```python
from build123d import *

# Parameters (mm, degrees)
EXTRUDE_1_DEPTH     = 5
CUT_EXTRUDE_1_REACH = 82.779
SKETCH_2_R          = 1.5


with BuildPart() as part:
    # 草图1 → 凸台-拉伸1 (new body)
    with BuildSketch(Plane(origin=(0, 0, 0), x_dir=(1, 0, 0), z_dir=(0, 1, 0))):
        with BuildLine():
            Line((61.023746461, 33.569203074), (60.837080184, 37.600567015))
            Line((60.837080184, 37.600567015), (70.826313722, 38.06310353))
            Line((70.826313722, 38.06310353), (71.011329506, 34.067384676))
            ThreePointArc((71.011329506, 34.067384676), (49.082411457, -9.842070835), (0.164945446, -13.841976975))
            ThreePointArc((0.164945446, -13.841976975), (-2.286053035, -7.209284728), (4.346639213, -4.758286247))
            ThreePointArc((4.346639213, -4.758286247), (43.480612021, -1.558361335), (61.023746461, 33.569203074))
        make_face()
    extrude(amount=EXTRUDE_1_DEPTH)

    # 草图2 → 切除-拉伸1 (cut, up to next)
    with BuildSketch(Plane(origin=(0, 5, 0), x_dir=(1, 0, 0), z_dir=(0, 1, 0)), mode=Mode.PRIVATE) as cut_extrude_1_sk1:
        with Locations(Location((16.930413815, -13.232401329, 0), (0, 0, 270))):
            Circle(SKETCH_2_R)
    cut_extrude_1_tool1 = extrude(cut_extrude_1_sk1.sketch, amount=-CUT_EXTRUDE_1_REACH, mode=Mode.PRIVATE) & part.part
    # 草图2 → 切除-拉伸1 (cut, up to next)
    with BuildSketch(Plane(origin=(0, 5, 0), x_dir=(1, 0, 0), z_dir=(0, 1, 0)), mode=Mode.PRIVATE) as cut_extrude_1_sk2:
        with Locations(Location((41.522785914, -8.508722595, 0), (0, 0, 270))):
            Circle(SKETCH_2_R)
    cut_extrude_1_tool2 = extrude(cut_extrude_1_sk2.sketch, amount=-CUT_EXTRUDE_1_REACH, mode=Mode.PRIVATE) & part.part
    add(cut_extrude_1_tool1.solids().sort_by_distance((16.930414, 5, 13.232401))[0], mode=Mode.SUBTRACT)
    add(cut_extrude_1_tool2.solids().sort_by_distance((41.522786, 5, 8.508723))[0], mode=Mode.SUBTRACT)


solid = part.part
```
Input: part model. Units: mm. Frame: model coordinates. A direction names the side the tool comes from. Give positions to 0.01 mm unless a question says otherwise; leave off trailing zeros. Order: outer loops, then holes, each group sorted by start corner. A loop starts at its lowest first (then second) coordinate and runs counter-clockwise, first axis right, second up. Notation, with made-up numbers: (-36.5, 27.25) - (12.5, 27.25) arc R16 ccw to (12.5, 33.25) - close; hole circle Ø11 at (13, 58.25). An arc over 180 degrees is marked (long way). Use a Markdown table: item, result.
(1) Section query A-A (y = 3.85). Output: boundary loops of the cut face in (x, z).
Computed values:
| item | result |
|---|---|
| outline | (0.16, 13.84) arc R5 ccw to (4.35, 4.76) arc R40 cw to (61.02, -33.57) - (60.84, -37.6) - (70.83, -38.06) - (71.01, -34.07) arc R50 ccw to start; hole circle Ø3 at (16.93, 13.23); hole circle Ø3 at (41.52, 8.51) |
(2) Draft query along X for faces 1 (the flat face through (45, 5, 1)), 2 (the cylindrical face through (18.195, 2.535, 14.039)), 3 (the flat face through (65.76, 2.46, -37.83)). Return one class per face: released by +X, released by -X, zero draft, split by the parting line, or undercut.
Computed values:
| item | result |
|---|---|
| face 1 | zero draft |
| face 2 | undercut |
| face 3 | released by -X |
(3) Pin query (flat end, axial travel): pin 1 (2 mm diameter, centred on x = 27, y = 1, fed in from +Z). Return the tip coordinate at first contact, or that it passes through.
Computed values:
| item | result |
|---|---|
| pin 1 | stops at z = 18.18 |
(4) Section query B-B (z = 1.5). Output: boundary loops of the cut face in (x, y), then the cut area to 3 significant figures.
Computed values:
| item | result |
|---|---|
| outline | (43.57, 0) - (58.57, 0) - (58.57, 5) - (43.57, 5) - close |
| area | 75.0 mm2 |
(5) Access query for faces 4 (the flat face through (70.918, 2.465, -36.093)), 5 (the flat face through (60.93, 2.46, -35.56)). Directions: +Z, -Z, +X, -X, +Y, -Y. A direction counts if a zero-diameter tool reaches every point of the face in a straight line with its end or side. Return the directions, or none.
Computed values:
| item | result |
|---|---|
| face 4 | -Z, +X, +Y, -Y |
| face 5 | -X, +Y, -Y |
(6) Section query C-C (x = 7). Output: boundary loops of the cut face in (y, z), then the cut area to 3 significant figures.
Computed values:
| item | result |
|---|---|
| outline | (0, 5.87) - (5, 5.87) - (5, 16.4) - (0, 16.4) - close |
| area | 52.7 mm2 |
(7) Line query: line 1 (Z direction, x = 18, y = 1.7); line 2 (Z direction, x = 21, y = 0.5); line 3 (X direction, y = 1.45, z = -32). Output: solid intervals per line, ascending. Write a range as from..to.
Computed values:
| item | result |
|---|---|
| line 1 | z = 8.31..12.18, 14.28..18.33 |
| line 2 | z = 8.42..18.42 |
| line 3 | x = 61.07..71.07 |
